Read the model definition and answer for the solid it produces. Units are mm, in the model's axes. A direction names the side the tool comes from. Coordinates: 2 decimals unless noted, no trailing zeros. Write each loop counter-clockwise with the first axis right and the second up, starting at its lowest first coordinate (ties: lowest second). Pieces come first, ordered by that corner, then holes.
(1) Which of the six approach directions +Z, -Z, +X, -X, +Y, -Y give full straight-line access (tool end or side, diameter ignored) to faces 1 (the flat face through (0, 27.2, 7)), 2 (the flat face through (25, 3, 1)), 3 (the flat face through (13, 2, 1)), 4 (the cylindrical face through (-11.63, -16.08, 9.99)), 5 (the flat face through (15.9, -2, 9.4))?
(2) Section B-B on z = 7 is taken. Write down the section's boundary in (x, y), then the cut area to 3 significant figures.
(3) Section C-C on x = -0.5 is taken. Write down the section's boundary in (y, z).
(4) Section A-A on y = 15 is taken. Write down the section's boundary in (x, z).
(5) The mould has two halves that part along Z. Classify faces 6 (the cylindrical face through (12.435, 28.58, 13.146)), 7 (the flat face through (0, 4, 11)), 8 (the cylindrical face through (-13.565, 28.58, 13.146)), 9 (the cylindrical face through (-12.872, 17.246, 9.986)): +Z half, -Z half, draft (parallel to the pull), parting line (faces both ways), or undercut.
(6) Section D-D on x = -20 is taken. Write down the section's boundary in (y, z).
(7) Given pin 1 (4 mm diameter, centred on x = 15, z = 7, fed in from -Y); pin 2 (6 mm diameter, centred on y = 19, z = 11, fed in from -X); pin 3 (9 mm diameter, centred on x = -2.5, y = -7.5, fed in from +Z); pin 4 (2 mm diameter, centred on x = -15.5, z = 5.5, fed in from +Y), each flat-ended and moving along its own axis, determine where each tip first touches the part or whether it passes through.
(8) Find the intervals of material crossed by probe 1 along X at (y, z) = (29.4, 13.7); probe 2 along X at (y, z) = (-17.95, 7); probe 3 along Y at (x, z) = (2, 4.5), in increasing order.
from build123d import *
from build123d.topology import SkipClean

# Parameters (mm, degrees)
SKETCH_1_W            = 57
SKETCH_1_H            = 51
SKETCH_1_W_2          = 3.4
SKETCH_1_H_2          = 3.4
SKETCH_1_W_3          = 7
SKETCH_1_H_3          = 42
EXTRUDE_1_DEPTH       = 3
SKETCH_2_W            = 31
SKETCH_2_H            = 47
CUT_EXTRUDE_1_DEPTH   = 1
SKETCH_5_W            = 57
SKETCH_5_H            = 3
EXTRUDE_2_DEPTH       = 1
SKETCH_6_W            = 57
SKETCH_6_H            = 3
EXTRUDE_3_DEPTH       = 1
SKETCH_7_W            = 10
SKETCH_7_H            = 3
EXTRUDE_4_DEPTH       = 6
SKETCH_8_W            = 31
SKETCH_8_H            = 3
EXTRUDE_5_DEPTH       = 6
CUT_EXTRUDE_3_REACH   = 63.082
SKETCH_9_R            = 1.15
EXTRUDE_6_OUTLINE_W   = 57
EXTRUDE_6_OUTLINE_H   = 53
EXTRUDE_6_OUTLINE_W_2 = 3.4
EXTRUDE_6_OUTLINE_H_2 = 3.4
EXTRUDE_6_OUTLINE_W_3 = 7
EXTRUDE_6_OUTLINE_H_3 = 42
EXTRUDE_6_DEPTH       = 0.5
EXTRUDE_7_DEPTH       = 0.2
EXTRUDE_START         = 0.2
SKETCH_14_R           = 1.15
EXTRUDE_8_DEPTH       = 0.2
CUT_EXTRUDE_START     = -0.2
SKETCH_15_R           = 1.15
CUT_EXTRUDE_5_DEPTH   = 0.2
CUT_EXTRUDE_6_DEPTH   = 0.2
SKETCH_17_W           = 31
SKETCH_17_H           = 3
EXTRUDE_9_DEPTH       = 5
SKETCH_18_W           = 31
SKETCH_18_H           = 2
EXTRUDE_10_DEPTH      = 50.4
SKETCH_3_R            = 1.25
CUT_EXTRUDE_7_DEPTH   = 9
EXTRUDE_START_2       = -0.2
EXTRUDE_11_OUTLINE_R  = 1.15
EXTRUDE_11_DEPTH      = 3.2
SKETCH_22_W           = 31
SKETCH_22_H           = 6
CUT_EXTRUDE_10_DEPTH  = 3
SKETCH_17_2_W         = 31
SKETCH_17_2_H         = 3
EXTRUDE_12_DEPTH      = 7.2
SKETCH_24_W           = 31
SKETCH_24_H           = 2
CUT_EXTRUDE_11_DEPTH  = 3
SKETCH_25_R           = 1.2
CUT_EXTRUDE_12_DEPTH  = 3
SKETCH_27_W           = 11
SKETCH_27_H           = 3.2
EXTRUDE_13_DEPTH      = 6
CUT_EXTRUDE_13_REACH  = 45.42
SKETCH_28_W           = 5
SKETCH_28_H           = 5
SKETCH_31_W           = 64.96263637
SKETCH_31_H           = 23.079945777
CUT_EXTRUDE_14_DEPTH  = 0.2
SKETCH_32_W           = 57
SKETCH_32_H           = 3.5
EXTRUDE_14_DEPTH      = 0.2
CUT_EXTRUDE_15_DEPTH  = 0.1
CUT_EXTRUDE_16_DEPTH  = 0.1


# Read off the part's stored shape, not the designer's step: 凸台-拉伸6, 凸台-拉伸11
with BuildPart() as part:
    # 草图1 → 凸台-拉伸1 (new body)
    with BuildSketch(Plane.XY):
        with Locations((0.5, 3.5)):
            Rectangle(SKETCH_1_W, SKETCH_1_H)
        with Locations((13.3, 0.3)):
            Rectangle(SKETCH_1_W_2, SKETCH_1_H_2, mode=Mode.SUBTRACT)
        with Locations((21.5, 3.5)):
            Rectangle(SKETCH_1_W_3, SKETCH_1_H_3, mode=Mode.SUBTRACT)
        with Locations((-20.5, 3.5)):
            Rectangle(SKETCH_1_W_3, SKETCH_1_H_3, mode=Mode.SUBTRACT)
    extrude(amount=EXTRUDE_1_DEPTH)

    # 草图2 → 切除-拉伸1 (cut)
    with BuildSketch(Plane.XY.offset(3)):
        with Locations((0.5, 3.5)):
            Rectangle(SKETCH_2_W, SKETCH_2_H)
    extrude(amount=-CUT_EXTRUDE_1_DEPTH, mode=Mode.SUBTRACT)

    # 草图5 → 凸台-拉伸2 (add)
    with BuildSketch(Plane(origin=(0, 29, 0), x_dir=(1, 0, 0), z_dir=(0, 1, 0))):
        with Locations((0.5, -1.5)):
            Rectangle(SKETCH_5_W, SKETCH_5_H)
    extrude(amount=EXTRUDE_2_DEPTH)

    # 草图6 → 凸台-拉伸3 (add)
    with BuildSketch(Plane(origin=(0, -22, 0), x_dir=(-1, 0, 0), z_dir=(0, -1, 0))):
        with Locations((-0.5, -1.5)):
            Rectangle(SKETCH_6_W, SKETCH_6_H)
    extrude(amount=EXTRUDE_3_DEPTH)

    # 草图7 → 凸台-拉伸4 (add)
    with BuildSketch(Plane.XY.offset(3)):
        with Locations((-10, -21.5)):
            Rectangle(SKETCH_7_W, SKETCH_7_H)
        with Locations((11, -21.5)):
            Rectangle(SKETCH_7_W, SKETCH_7_H)
    extrude(amount=EXTRUDE_4_DEPTH)

    # 草图8 → 凸台-拉伸5 (add)
    with BuildSketch(Plane.XY.offset(3)):
        with Locations((0.5, 28.5)):
            Rectangle(SKETCH_8_W, SKETCH_8_H)
    extrude(amount=EXTRUDE_5_DEPTH)

    # 草图9 → 切除-拉伸3 (cut, up to next)
    with BuildSketch(Plane.XZ.offset(23), mode=Mode.PRIVATE) as cut_extrude_3_sk1:
        with Locations(Location((-10, 7, 0), (0, 0, 270))):
            Circle(SKETCH_9_R)
    cut_extrude_3_tool1 = extrude(cut_extrude_3_sk1.sketch, amount=-CUT_EXTRUDE_3_REACH, mode=Mode.PRIVATE) & part.part
    # 草图9 → 切除-拉伸3 (cut, up to next)
    with BuildSketch(Plane.XZ.offset(23), mode=Mode.PRIVATE) as cut_extrude_3_sk2:
        with Locations(Location((11, 7, 0), (0, 0, 270))):
            Circle(SKETCH_9_R)
    cut_extrude_3_tool2 = extrude(cut_extrude_3_sk2.sketch, amount=-CUT_EXTRUDE_3_REACH, mode=Mode.PRIVATE) & part.part
    add(cut_extrude_3_tool1.solids().sort_by_distance((-10, -23, 7))[0], mode=Mode.SUBTRACT)
    add(cut_extrude_3_tool2.solids().sort_by_distance((11, -23, 7))[0], mode=Mode.SUBTRACT)

    # 凸台-拉伸6 outline → 凸台-拉伸6 (add)
    with BuildSketch(Plane(origin=(0, 0, 0), x_dir=(-1, 0, 0), z_dir=(0, 0, -1))):
        with Locations((-0.5, 3.5)):
            Rectangle(EXTRUDE_6_OUTLINE_W, EXTRUDE_6_OUTLINE_H)
        with Locations((-13.3, 0.3)):
            Rectangle(EXTRUDE_6_OUTLINE_W_2, EXTRUDE_6_OUTLINE_H_2, mode=Mode.SUBTRACT)
        with Locations((-21.5, 3.5)):
            Rectangle(EXTRUDE_6_OUTLINE_W_3, EXTRUDE_6_OUTLINE_H_3, mode=Mode.SUBTRACT)
        with Locations((20.5, 3.5)):
            Rectangle(EXTRUDE_6_OUTLINE_W_3, EXTRUDE_6_OUTLINE_H_3, mode=Mode.SUBTRACT)
    extrude(amount=EXTRUDE_6_DEPTH)

    # 草图13 → 凸台-拉伸7 (add)
    with BuildSketch(Plane(origin=(0, 30, 0), x_dir=(1, 0, 0), z_dir=(0, 1, 0))):
        Polygon((16, -3), (29, -3), (29, 0.5), (-28, 0.5), (-28, -3), (-15, -3), (-15, -9), (16, -9), align=None)
    extrude(amount=EXTRUDE_7_DEPTH)

    # 草图14 → 凸台-拉伸8 (add)
    with BuildSketch(Plane(origin=(0, -23, 0), x_dir=(-1, 0, 0), z_dir=(0, -1, 0)).offset(EXTRUDE_START)):
        Polygon((-29, 0.5), (-29, -3), (-16, -3), (-16, -9), (-6, -9), (-6, -3), (5, -3), (5, -9), (15, -9), (15, -3), (28, -3), (28, 0.5), align=None)
        with Locations(Location((-11, -7, 0), (0, 0, 90))):
            Circle(SKETCH_14_R, mode=Mode.SUBTRACT)
        with Locations(Location((10, -7, 0), (0, 0, 90))):
            Circle(SKETCH_14_R, mode=Mode.SUBTRACT)
    extrude(amount=-EXTRUDE_8_DEPTH)

    # 草图15 → 切除-拉伸5 (cut)
    with BuildSketch(Plane(origin=(0, -20, 0), x_dir=(1, 0, 0), z_dir=(0, 1, 0)).offset(CUT_EXTRUDE_START)):
        Polygon((16, -2), (-15, -2), (-15, -3), (-15, -9), (-5, -9), (-5, -3), (6, -3), (6, -9), (16, -9), (16, -3), align=None)
        with Locations(Location((11, -7, 0), (0, 0, 90))):
            Circle(SKETCH_15_R, mode=Mode.SUBTRACT)
        with Locations(Location((-10, -7, 0), (0, 0, 90))):
            Circle(SKETCH_15_R, mode=Mode.SUBTRACT)
    extrude(amount=CUT_EXTRUDE_5_DEPTH, mode=Mode.SUBTRACT)

    # 草图16 → 切除-拉伸6 (cut)
    with BuildSketch(Plane.XZ.offset(-27)):
        Polygon((-15, 2), (16, 2), (16, 3), (16, 9), (-15, 9), (-15, 3), align=None)
    extrude(amount=-CUT_EXTRUDE_6_DEPTH, mode=Mode.SUBTRACT)

    # 草图17 → 凸台-拉伸9 (add)
    with BuildSketch(Plane.XY.offset(9)):
        with Locations((0.5, 28.7)):
            Rectangle(SKETCH_17_W, SKETCH_17_H)
    extrude(amount=EXTRUDE_9_DEPTH)

    # 草图18 → 凸台-拉伸10 (add)
    with BuildSketch(Plane.XZ.offset(-27.2)):
        with Locations((0.5, 10)):
            Rectangle(SKETCH_18_W, SKETCH_18_H)
    extrude(amount=EXTRUDE_10_DEPTH)

    # 草图3 → 切除-拉伸7 (cut)
    with BuildSketch(Plane.XY.offset(2)):
        with Locations(Location((-12.2, 18.3, 0), (0, 0, 180))):
            Circle(SKETCH_3_R)
        with Locations(Location((13.2, 18.1, 0), (0, 0, 180))):
            Circle(SKETCH_3_R)
        with Locations(Location((12.9, -17.3, 0), (0, 0, 180))):
            Circle(SKETCH_3_R)
        with Locations(Location((-11.9, -17.3, 0), (0, 0, 180))):
            Circle(SKETCH_3_R)
    extrude(amount=CUT_EXTRUDE_7_DEPTH, mode=Mode.SUBTRACT)

    # 凸台-拉伸11 outline → 凸台-拉伸11 (add)
    with SkipClean():  # the faces are left unmerged after this step: merging them gives an invalid solid
        with BuildSketch(Plane(origin=(0, -20, 0), x_dir=(1, 0, 0), z_dir=(0, 1, 0)).offset(EXTRUDE_START_2)):
            Polygon((-5, -9), (-5, -3), (6, -3), (6, -9), (16, -9), (16, -2), (-15, -2), (-15, -9), align=None)
            with Locations((-10, -7)):
                Circle(EXTRUDE_11_OUTLINE_R, mode=Mode.SUBTRACT)
            with Locations((11, -7)):
                Circle(EXTRUDE_11_OUTLINE_R, mode=Mode.SUBTRACT)
        extrude(amount=EXTRUDE_11_DEPTH)

    # 草图22 → 切除-拉伸10 (cut)
    with BuildSketch(Plane(origin=(0, -23.2, 0), x_dir=(-1, 0, 0), z_dir=(0, -1, 0))):
        with Locations((-0.5, -6)):
            Rectangle(SKETCH_22_W, SKETCH_22_H)
    extrude(amount=-CUT_EXTRUDE_10_DEPTH, mode=Mode.SUBTRACT)

    # 草图17<2> → 凸台-拉伸12 (add)
    with BuildSketch(Plane.XY.offset(9)):
        with Locations((0.5, 28.7)):
            Rectangle(SKETCH_17_2_W, SKETCH_17_2_H)
    extrude(amount=EXTRUDE_12_DEPTH)

    # 草图24 → 切除-拉伸11 (cut)
    with BuildSketch(Plane.XZ.offset(23.2)):
        with Locations((0.5, 10)):
            Rectangle(SKETCH_24_W, SKETCH_24_H)
    extrude(amount=-CUT_EXTRUDE_11_DEPTH, mode=Mode.SUBTRACT)

    # 草图25 → 切除-拉伸12 (cut)
    with BuildSketch(Plane.XZ.offset(-27.2)):
        with Locations(Location((-12.5, 13.7, 0), (0, 0, 270))):
            Circle(SKETCH_25_R)
        with Locations(Location((13.5, 13.7, 0), (0, 0, 270))):
            Circle(SKETCH_25_R)
    extrude(amount=-CUT_EXTRUDE_12_DEPTH, mode=Mode.SUBTRACT)

    # 草图27 → 凸台-拉伸13 (add)
    with BuildSketch(Plane.XY.offset(3)):
        with Locations((0.5, -18.6)):
            Rectangle(SKETCH_27_W, SKETCH_27_H)
    extrude(amount=EXTRUDE_13_DEPTH)

    # 草图28 → 切除-拉伸13 (cut, up to next)
    with BuildSketch(Plane.XY.offset(11), mode=Mode.PRIVATE) as cut_extrude_13_sk1:
        with Locations((13.5, 24.7)):
            Rectangle(SKETCH_28_W, SKETCH_28_H)
    cut_extrude_13_tool1 = extrude(cut_extrude_13_sk1.sketch, amount=-CUT_EXTRUDE_13_REACH, mode=Mode.PRIVATE) & part.part
    add(cut_extrude_13_tool1.solids().sort_by_distance((13.5, 24.7, 11))[0], mode=Mode.SUBTRACT)

    # 草图31 → 切除-拉伸14 (cut)
    with BuildSketch(Plane(origin=(0, 30.2, 0), x_dir=(1, 0, 0), z_dir=(0, 1, 0))):
        with Locations((-0.558713109, -6.113710501)):
            Rectangle(SKETCH_31_W, SKETCH_31_H)
    extrude(amount=-CUT_EXTRUDE_14_DEPTH, mode=Mode.SUBTRACT)

    # 草图32 → 凸台-拉伸14 (add)
    with BuildSketch(Plane.XZ.offset(23.2)):
        with Locations((0.5, 1.25)):
            Rectangle(SKETCH_32_W, SKETCH_32_H)
    extrude(amount=EXTRUDE_14_DEPTH)

    # 草图33 → 切除-拉伸15 (cut)
    with BuildSketch(Plane.ZY.offset(15)):
        Polygon((16.2, 27.2), (16.2, 30), (3, 30), (3, 27.2), (9, 27.2), (9, -17), (3, -17), (3, -20.2), (11, -20.2), (11, 27.2), align=None)
    extrude(amount=-CUT_EXTRUDE_15_DEPTH, mode=Mode.SUBTRACT)

    # 草图34 → 切除-拉伸16 (cut)
    with BuildSketch(Plane(origin=(16, 0, 0), x_dir=(0, 0, -1), z_dir=(1, 0, 0))):
        Polygon((-3, -17), (-9, -17), (-9, 22.2), (-11, 22.2), (-11, -20.2), (-3, -20.2), align=None)
    extrude(amount=-CUT_EXTRUDE_16_DEPTH, mode=Mode.SUBTRACT)


solid = part.part
Response:
1. face 1: none
1. face 2: +Z, -Z
1. face 3: -Z
1. face 4: +Z
1. face 5: +Z, +X, -Y
2. outline: (-14.9, -20.2) - (-11.15, -20.2) - (-11.15, -17) - (-14.9, -17) - close; (-14.9, 27.2) - (16, 27.2) - (16, 30) - (-14.9, 30) - close; (-8.85, -20.2) - (9.85, -20.2) - (9.85, -17) - (-8.85, -17) - close; (12.15, -20.2) - (15.9, -20.2) - (15.9, -17) - (12.15, -17) - close
2. area: 170 mm2
3. outline: (-23.4, -0.5) - (30, -0.5) - (30, 16.2) - (27.2, 16.2) - (27.2, 11) - (-20.2, 11) - (-20.2, 3) - (-23.4, 3) - close; hole (-17, 2) - (27.2, 2) - (27.2, 9) - (-17, 9) - close
4. outline: (-28, -0.5) - (-24, -0.5) - (-24, 3) - (-28, 3) - close; (-17, -0.5) - (18, -0.5) - (18, 3) - (16, 3) - (16, 2) - (-15, 2) - (-15, 3) - (-17, 3) - close; (-14.9, 9) - (15.9, 9) - (15.9, 11) - (-14.9, 11) - close; (25, -0.5) - (29, -0.5) - (29, 3) - (25, 3) - close
5. face 6: undercut
5. face 7: +Z half
5. face 8: undercut
5. face 9: draft
6. outline: (-23.4, -0.5) - (-17.5, -0.5) - (-17.5, 3) - (-23.4, 3) - close; (24.5, -0.5) - (30, -0.5) - (30, 3) - (24.5, 3) - close
7. pin 1: stops at y = -20.2
7. pin 2: stops at x = -14.9
7. pin 3: stops at z = 11
7. pin 4: stops at y = 30
8. probe 1: x = -14.9 to -13.7, -11.3 to 12.3, 14.7 to 16
8. probe 2: x = -14.9 to -11.15, -8.85 to 9.85, 12.15 to 15.9
8. probe 3: y = -20.2 to -17, 27.2 to 30
